Here's how the part is built. I have some questions about the finished solid (model axes, mm). A direction names the side the tool comes from. Give positions to 0.01 mm unless a question says otherwise; leave off trailing zeros. Loops run counter-clockwise (first coordinate to the right, second up) from the corner with the lowest first, then second, coordinate; pieces in that order, holes last.
Q1. If we section it at A-A (x = 31): Please give me the cut outline in (y, z).
Q2. We'd pull the mould along X, two halves only. Please class faces 1 (the face through (43.9, 0, 23.4)), 2 (the face through (44.574, 1.676, -21.404)), 3 (the face through (62, 0.3, -0.4)), 4 (the face through (43, 0, 0)): +X half, -X half, draft (parallel to the pull), parting line (faces both ways), or undercut.
Q3. If we section it at D-D (x = 41.5): Please give me the cut outline in (y, z), plus the area to 3 significant figures.
Q4. If we section it at C-C (y = -2): Please give me the cut outline in (x, z), plus the area to 3 significant figures.
Q5. Will these pins go through, and if not, where does the flat tip stop? P1, Ø5.5, axis at x = 43, z = -20, coming from the -Y side; P2, Ø3, axis at x = 56, z = 0, coming from the -Y side.
Q6. I need wall thicknesses on line 1 (X direction, y = 2.15, z = 0); line 2 (Z direction, x = 30.5, y = -6.75); line 3 (X direction, y = -4.5, z = -21). Which ranges of each line are inside material? Lowest first, please.
Q7. For faces 5 (the face through (43, -4, -6.55)), 6 (the face through (47, -8.1, 18)), 7 (the face through (43.9, 0, -18.6)), which set-ups out of +Z, -Z, +X, -X, +Y, -Y let a thin tool reach every point of the face, with its end or its side?
Q8. If we section it at B-B (z = -21): Please give me the cut outline in (x, y).
from build123d import *

# Parameters (mm, degrees)
SKETCH7_W            = 37
SKETCH7_H            = 60
SKETCH7_R            = 3.1
SKETCH7_R_2          = 2
BOSS_EXTRUDE10_DEPTH = 3.4
SKETCH8_W            = 37
SKETCH8_H            = 23.45
SKETCH8_R            = 5.5
BOSS_EXTRUDE12_DEPTH = 8.1


with BuildPart() as part:
    # Sketch7 → Boss-Extrude10 (new body)
    with BuildSketch(Plane(origin=(0, 0, 0), x_dir=(1, 0, 0), z_dir=(0, 1, 0))):
        with Locations((43.5, 0)):
            Rectangle(SKETCH7_W, SKETCH7_H)
        with Locations(Location((41.5, 21, 0), (0, 0, 270))):
            Circle(SKETCH7_R, mode=Mode.SUBTRACT)
        with Locations(Location((41.5, -21, 0), (0, 0, 90))):
            Circle(SKETCH7_R, mode=Mode.SUBTRACT)
        with Locations(Location((56, 0, 0), (0, 0, 270))):
            Circle(SKETCH7_R_2, mode=Mode.SUBTRACT)
        with Locations(Location((31, 0, 0), (0, 0, 270))):
            Circle(SKETCH7_R_2, mode=Mode.SUBTRACT)
    extrude(amount=BOSS_EXTRUDE10_DEPTH)

    # Sketch8 → Boss-Extrude12 (add)
    # profile 1 of 2: a face of its own
    with BuildSketch(Plane.XZ):
        with Locations((43.5, 18.275)):
            Rectangle(SKETCH8_W, SKETCH8_H)
        with Locations(Location((41.5, 21, 0), (0, 0, 270))):
            Circle(SKETCH8_R, mode=Mode.SUBTRACT)
    # profile 2 of 2: a face of its own
    with BuildSketch(Plane.XZ):
        with Locations((43.5, -18.275)):
            Rectangle(SKETCH8_W, SKETCH8_H)
        with Locations(Location((41.5, -21, 0), (0, 0, 90))):
            Circle(SKETCH8_R, mode=Mode.SUBTRACT)
    extrude(amount=BOSS_EXTRUDE12_DEPTH)


solid = part.part
Check sheet entries:
1. outline: (-8.1, -30) - (3.4, -30) - (3.4, -2) - (0, -2) - (0, -6.55) - (-8.1, -6.55) - close; (-8.1, 6.55) - (0, 6.55) - (0, 2) - (3.4, 2) - (3.4, 30) - (-8.1, 30) - close
2. face 1: undercut
2. face 2: undercut
2. face 3: +X half
2. face 4: draft
3. outline: (-8.1, -30) - (3.4, -30) - (3.4, -24.1) - (0, -24.1) - (0, -26.5) - (-8.1, -26.5) - close; (-8.1, -15.5) - (0, -15.5) - (0, -17.9) - (3.4, -17.9) - (3.4, 17.9) - (0, 17.9) - (0, 15.5) - (-8.1, 15.5) - (-8.1, 6.55) - (0, 6.55) - (0, -6.55) - (-8.1, -6.55) - close; (-8.1, 26.5) - (0, 26.5) - (0, 24.1) - (3.4, 24.1) - (3.4, 30) - (-8.1, 30) - close
3. area: 364 mm2
4. outline: (25, -30) - (62, -30) - (62, -6.55) - (25, -6.55) - close; (25, 6.55) - (62, 6.55) - (62, 30) - (25, 30) - close; hole circle Ø11 at (41.5, -21); hole circle Ø11 at (41.5, 21)
4. area: 1,550 mm2
5. P1: stops at y = 0
5. P2: passes through
6. line 1: x = 25 to 29, 33 to 54, 58 to 62
6. line 2: z = -30 to -6.55, 6.55 to 30
6. line 3: x = 25 to 36, 47 to 62
7. face 5: +X, -X, -Y
7. face 6: +Z, -Z, +X, -X, -Y
7. face 7: -Y
8. outline: (25, -8.1) - (36, -8.1) - (36, 0) - (38.4, 0) - (38.4, 3.4) - (25, 3.4) - close; (44.6, 0) - (47, 0) - (47, -8.1) - (62, -8.1) - (62, 3.4) - (44.6, 3.4) - close
